Verification items for the finished model (mm, model axes). A direction names the side the tool comes from. Coordinates: 2 decimals unless noted, no trailing zeros. Order: outer loops, then holes, each group sorted by start corner. A loop starts at its lowest first (then second) coordinate and runs counter-clockwise, first axis right, second up. Notation, with made-up numbers: M 70.25,76.25 L 116.25,76.25 A14 ccw 116.25,96.25 Z; hole C -20.5,-13 d8. An arc over 180 degrees is marked long. Return JSON: item names as keys, results as strings. Group by question number.
Q1. Section check D-D, the plane y = 3.35. Enter the section's corners in (x, z), then the cut area to 3 significant figures.
Q2. Thickness scan on probe 1 along Y at (x, z) = (-2.25, 4.5); probe 2 along Y at (x, z) = (-0.75, -2); probe 3 along Z at (x, y) = (0, 2.95). Record the ranges inside material, lowest first.
Q3. Access from +Z, -Z, +X, -X, +Y, -Y to the whole of each face (thin tool, end or side, straight path). Record for faces 1 (the face through (-1, 2, 1)), 2 (the face through (1.29, 0.493, 2.024)), 3 (the face through (0.7, 4, 2.3)).
Q4. Section check A-A, the plane y = 1.25. Enter the section's corners in (x, z), then the cut area to 3 significant figures.
Q5. Go/stop test with flat-tipped pins: pin 1 Ø2 at (y, z) = (2, 8) entering from -X; pin 2 Ø3.5 at (x, z) = (0, 0) entering from +Y; pin 3 Ø1.6 at (x, z) = (0, 0) entering from +Y; pin 4 Ø1.5 at (x, y) = (1.5, 2) entering from +Z. Record where each tip stops, or that it passes through.
Q6. Section check B-B, the plane z = 9. Enter the section's corners in (x, y).
Q7. Mould release check, pull along Z, two halves, no side actions. Record for faces 4 (the face through (-1, 0, 7)), 5 (the face through (-0.29, 3.01, -2.23)), 6 (the face through (0.066, 1.604, 0.998)), 7 (the face through (0, 1, 17)): pulls with the +Z half, pulls with the -Z half, needs draft (parallel to the pull), parting line crosses it, or undercut.
Autodesk Inventor part; units mm, degrees
ref_plane "YZ Plane" through (0, 0, 0) normal (1, 0, 0) x (0, 1, 0)
ref_plane "XZ Plane" through (0, 0, 0) normal (0, 1, 0) x (-1, 0, 0)
ref_plane "XY Plane" through (0, 0, 0) normal (0, 0, 1) x (1, 0, 0)
sketch "Эскиз1" plane through (0, 0, 0) normal (0, 1, 0) x (-1, 0, 0)
  circle A0 centre (0, 0) radius 1
  circle A1 centre (0, 0) radius 3.5
  arc A2 (1.9956, 15.1325) -> (-1.9956, 15.1325) centre (0, 15) ccw
  line L0 (1.9956, 15.1325) -> (2.8667, 2.008)
  line L1 (-1.9956, 15.1325) -> (-2.8667, 2.008)
  circle A3 centre (0, 15) radius 0.25
  circle A4 centre (0, 13) radius 0.25
  circle A5 centre (0, 11) radius 0.25
  circle A6 centre (0, 9) radius 0.25
  circle A7 centre (0, 7) radius 0.25
  circle A8 centre (0, 5) radius 0.25
  line L2 (2.8667, 2.008) -> (3, 0) construction
  line L3 (-2.8667, 2.008) -> (-3, 0) construction
  dimension "d0" = 7
  dimension "d1" = 2
  dimension "d2" = 3
  dimension "d3" = 3
  dimension "d4" = 15
  dimension "d5" = 2
  dimension "d6" = 0.5
  dimension "d7" = 0.5
  dimension "d8" = 0.5
  dimension "d9" = 0.5
  dimension "d10" = 0.5
  dimension "d11" = 0.5
  dimension "d13" = 2
  dimension "d14" = 2
  dimension "d15" = 2
  dimension "d16" = 2
  dimension "d17" = 2
extrude "Выдавливание1" add sketch "Эскиз1" along normal blind 1.5
sketch "Эскиз2" plane through (0, 1.5, 0) normal (0, 1, 0) x (1, 0, 0)
  arc A0 (2.8667, -2.008) -> (-2.8667, -2.008) centre (0, 0) ccw
  circle A1 centre (0, 0) radius 1
  circle A2 centre (0, 0) radius 3.5
extrude "Выдавливание2" add sketch "Эскиз2" along normal blind 2.5
sketch "Эскиз3" plane through (0, 4, 0) normal (0, 1, 0) x (1, 0, 0)
  circle A0 centre (0, 0) radius 1
  circle A1 centre (0, 0) radius 2.25
  dimension "d23" = 4.5
extrude "Выдавливание3" cut sketch "Эскиз3" against normal blind 2
sketch "Эскиз4" plane through (0, 0, 0) normal (0, -1, 0) x (1, 0, 0)
  circle A0 centre (0, 0) radius 2.4
  dimension "d29" = 4.8
extrude "Выдавливание4" cut sketch "Эскиз4" against normal blind 1
equation "\"d7\" = d6"
equation "\"d8\" = d6"
equation "\"d9\" = d6"
equation "\"d10\" = d6"
equation "\"d11\" = d6"
properties part number "Arm 1" material "Нейлон 6/6"
Numbers:
{
 "1": {"outline": "M -2.87,2.01 A3.5 ccw long 2.87,2.01 A3.5 ccw Z; hole C 0,0 d4.5", "area": "22.6 mm2"},
 "2": {"probe 1": "y = 0 to 1.5", "probe 2": "y = 1 to 2", "probe 3": "z = -3.5 to -2.25, 2.25 to 3.5"},
 "3": {"face 1": "+Y", "face 2": "-Y", "face 3": "+Z, -Z, +X, -X, +Y"},
 "4": {"outline": "M -2.87,2.01 A3.5 ccw long 2.87,2.01 L 2,15.13 A2 ccw -2,15.13 Z; hole C 0,0 d2; hole C 0,5 d0.5; hole C 0,7 d0.5; hole C 0,9 d0.5; hole C 0,11 d0.5; hole C 0,13 d0.5; hole C 0,15 d0.5", "area": "97.7 mm2"},
 "5": {"pin 1": "stops at x = -2.53", "pin 2": "stops at y = 2", "pin 3": "passes through", "pin 4": "stops at z = 16.76"},
 "6": {"outline": "M -2.4,0 L -0.25,0 L -0.25,1.5 L -2.4,1.5 Z; M 0.25,0 L 2.4,0 L 2.4,1.5 L 0.25,1.5 Z"},
 "7": {"face 4": "needs draft", "face 5": "undercut", "face 6": "undercut", "face 7": "pulls with the +Z half"}
}
